Build history of the part. All positions in model axes, mm. A direction names the side the tool comes from. Round coordinates to 2 decimals unless told otherwise and drop trailing zeros. Loops run counter-clockwise (first coordinate to the right, second up) from the corner with the lowest first, then second, coordinate; pieces in that order, holes last. Notation, with made-up numbers: M -28,-1 L 20,-1 A15 cw 20,14 Z; hole C -14,56 d5. An arc over 180 degrees is marked long. Use one line per item in the form item = value. Start each with the question number.
```python
from build123d import *

# Parameters (mm, degrees)
BOSS_EXTRUDE1_DEPTH = 6.35
FILLET1_R           = 1.524
FILLET2_R           = 3.5179
CUT_EXTRUDE1_REACH  = 36.405
SKETCH4_R           = 2.3495
CUT_EXTRUDE3_REACH  = 36.405
SKETCH6_R           = 2.3495
FILLET3_R           = 0.19939


with BuildPart() as part:
    # Sketch3 → Boss-Extrude1 (new, symmetric)
    with BuildSketch(Plane(origin=(0, 0, 0), x_dir=(1, 0, 0), z_dir=(0, 1, 0))):
        Polygon((0.99695, -24.40305), (-0.99695, -24.40305), (-0.99695, 0.99695), (24.40305, 0.99695), (24.40305, -0.99695), (0.99695, -0.99695), align=None)
    extrude(amount=BOSS_EXTRUDE1_DEPTH, both=True)

    # Fillet1
    fillet1_edges = [part.edges().sort_by_distance(p)[0] for p in [
        (0.99695, 0, 0.99695),
    ]]
    fillet(fillet1_edges, radius=FILLET1_R)

    # Fillet2
    fillet2_edges = [part.edges().sort_by_distance(p)[0] for p in [
        (-0.99695, 0, -0.99695),
    ]]
    fillet(fillet2_edges, radius=FILLET2_R)

    # Sketch4 → Cut-Extrude1 (cut, up to next)
    with BuildSketch(Plane.XY.offset(0.99695), mode=Mode.PRIVATE) as cut_extrude1_sk1:
        with Locations((14.75105, 0)):
            Circle(SKETCH4_R)
    cut_extrude1_tool1 = extrude(cut_extrude1_sk1.sketch, amount=-CUT_EXTRUDE1_REACH, mode=Mode.PRIVATE) & part.part
    add(cut_extrude1_tool1.solids().sort_by_distance((14.75105, 0, 0.99695))[0], mode=Mode.SUBTRACT)

    # Cut-Extrude2 cone 1 section (through the dimple's axis) → Cut-Extrude2 (revolve, cut)
    with BuildSketch(Plane(origin=(14.75105, 0, 0.99695), x_dir=(0, -1, 0), z_dir=(1, 0, 0))):
        Polygon((0, 0), (3.5433, 0), (0, 4.076100377), align=None)
    revolve(axis=Axis((14.75105, 0, 0.99695), (0, 0, -1)), mode=Mode.SUBTRACT)

    # Sketch6 → Cut-Extrude3 (cut, up to next)
    with BuildSketch(Plane(origin=(0.99695, 0, 0), x_dir=(0, 0, -1), z_dir=(1, 0, 0)), mode=Mode.PRIVATE) as cut_extrude3_sk1:
        with Locations((-14.75105, 0)):
            Circle(SKETCH6_R)
    cut_extrude3_tool1 = extrude(cut_extrude3_sk1.sketch, amount=-CUT_EXTRUDE3_REACH, mode=Mode.PRIVATE) & part.part
    add(cut_extrude3_tool1.solids().sort_by_distance((0.99695, 0, 14.75105))[0], mode=Mode.SUBTRACT)

    # Cut-Extrude4 cone 1 section (through the dimple's axis) → Cut-Extrude4 (revolve, cut)
    with BuildSketch(Plane(origin=(0.99695, 0, 14.75105), x_dir=(0, 0, -1), z_dir=(0, 1, 0))):
        Polygon((0, 0), (3.5433, 0), (0, 4.076100377), align=None)
    revolve(axis=Axis((0.99695, 0, 14.75105), (-1, 0, 0)), mode=Mode.SUBTRACT)

    # Fillet3
    fillet3_edges = [part.edges().sort_by_distance(p)[0] for p in [
        (0.99695, 6.35, 13.462),
        (24.40305, 0, -0.99695),
        (24.40305, 0, 0.99695),
        (0.99695, 0, 24.40305),
        (-0.99695, 0, 24.40305),
        (24.40305, 6.35, 0),
        (13.462, -6.35, 0.99695),
        (13.462, 6.35, 0.99695),
        (13.462, 6.35, -0.99695),
        (1.443319265, -6.35, 1.443319265),
        (1.443319265, 6.35, 1.443319265),
        (-0.99695, -6.35, 13.462),
        (-0.99695, 6.35, 13.462),
        (0.033419054, -6.35, 0.033419054),
        (0.033419054, 6.35, 0.033419054),
        (13.462, -6.35, -0.99695),
        (24.40305, -6.35, 0),
        (0, 6.35, 24.40305),
        (0.99695, -6.35, 13.462),
        (0, -6.35, 24.40305),
    ]]
    fillet(fillet3_edges, radius=FILLET3_R)


solid = part.part
```
Q1. Wall check: probe 1 along X at (y, z) = (0, -0.55); probe 2 along X at (y, z) = (-5.25, 17.25). Give the ranges that are in metal, low to high.
Q2. Pull direction Y, two halves, no side cores. Call faces 3 (the face through (24.403, 0, 0)), 4 (the face through (6.2, 6.35, 0.5)), 5 (the face through (-0.68, 1.59, 16.48)): pulls with the +Y half, pulls with the -Y half, needs draft (parallel to the pull), parting line crosses it, or undercut.
Q3. Drop flat-ended pins along their axis: P1, Ø6, axis at x = 9.5, y = 1, coming from the +Z side; P2, Ø5, axis at y = 2.5, z = 20.5, coming from the +X side; P3, Ø1.5, axis at y = -1, z = 14, coming from the -X side. Give the stop position or say it passes through.
Q4. Saw through at B-B (x = 4.25). Give the cut face in (y, z).
Q5. Saw through at C-C (y = -4.5). Give the cut face in (x, z).
Q6. Saw through at A-A (y = 0). Give the cut face in (x, z), and give its area (3 significant figures).
Q7. Tool access for faces 1 (the face through (11, 0, -0.997)), 2 (the face through (11, 0, 0.997)): list every direction of +Z, -Z, +X, -X, +Y, -Y with a clear straight run to the whole face (end or side of a thin tool).
Q8. Saw through at D-D (z = 3). Give the cut face in (x, y).
Filled in:
q1.probe_1 = 0.8 to 12.4, 17.1 to 24.4
q1.probe_2 = -1 to 1
q2.face_3 = needs draft
q2.face_4 = pulls with the +Y half
q2.face_5 = undercut
q3.P1 = 1
q3.P2 = 1
q3.P3 = through
q4.outline = M -6.35,-0.8 A0.2 ccw -6.15,-1 L 6.15,-1 A0.2 ccw 6.35,-0.8 L 6.35,0.8 A0.2 ccw 6.15,1 L -6.15,1 A0.2 ccw -6.35,0.8 Z
q5.outline = M -1,2.52 A3.52 ccw 2.52,-1 L 24.2,-1 A0.2 ccw 24.4,-0.8 L 24.4,0.8 A0.2 ccw 24.2,1 L 2.52,1 A1.52 cw 1,2.52 L 1,24.2 A0.2 ccw 0.8,24.4 L -0.8,24.4 A0.2 ccw -1,24.2 Z
q6.outline = M -1,2.52 A3.52 ccw 2.52,-1 L 12.4,-1 L 12.4,-0.38 L 11.21,1 L 2.52,1 A1.52 cw 1,2.52 L 1,11.21 L -0.38,12.4 L -1,12.4 Z; M -1,17.1 L -0.38,17.1 L 1,18.29 L 1,24.2 A0.2 ccw 0.8,24.4 L -0.8,24.4 A0.2 ccw -1,24.2 Z; M 17.1,-1 L 24.2,-1 A0.2 ccw 24.4,-0.8 L 24.4,0.8 A0.2 ccw 24.2,1 L 18.29,1 L 17.1,-0.38 Z
q6.area = 73.1 mm²
q7.face_1 = -Z, +X, -X, +Y, -Y
q7.face_2 = +Z, +X, +Y, -Y
q8.outline = M -1,-6.15 A0.2 ccw -0.8,-6.35 L 0.8,-6.35 A0.2 ccw 1,-6.15 L 1,6.15 A0.2 ccw 0.8,6.35 L -0.8,6.35 A0.2 ccw -1,6.15 Z
